```python
from build123d import *

# Parameters (mm, degrees)
BOSS_EXTRUDE2_DEPTH             = 6.896
SKETCH2_R                       = 1.7526
BOSS_EXTRUDE3_DEPTH             = 3.175
F_9_64_0_14063_DIAMETER_HOLE2_D = 3.572002
SKETCH9_W                       = 3.175
SKETCH9_H                       = 6.896
BOSS_EXTRUDE5_DEPTH             = 2.54
SKETCH10_W                      = 3.175
SKETCH10_H                      = 12.7
SKETCH10_W_2                    = 12.7
SKETCH10_H_2                    = 3.175
BOSS_EXTRUDE6_DEPTH             = 3.175
CUT_EXTRUDE1_DEPTH              = 97.085734956
CUT_EXTRUDE2_DEPTH              = 66.25004773
FILLET2_R                       = 1
CUT_EXTRUDE3_DEPTH              = 1


with BuildPart() as part:
    # Sketch1 → Boss-Extrude2 (new body)
    with BuildSketch(Plane(origin=(0, 0, 0), x_dir=(1, 0, 0), z_dir=(0, 1, 0))):
        with BuildLine():
            Line((12.363664128, -36.460798254), (6.35, -38.5))
            Line((6.35, -38.5), (-6.35, -38.5))
            Line((-6.35, -38.5), (-12.363664128, -36.460798254))
            ThreePointArc((-12.363664128, -36.460798254), (-27.097558937, -27.349082245), (-36.345013413, -12.7))
            ThreePointArc((-36.345013413, -12.7), (-37.940572846, -6.539337285), (-38.499480516, -0.2))
            Line((-38.499480516, -0.2), (-41.675, -0.2))
            Line((-41.675, -0.2), (-41.675, -15.875))
            Line((-41.675, -15.875), (-31.113215051, -27.726764582))
            ThreePointArc((-31.113215051, -27.726764582), (-23.009697223, -34.747078419), (-13.383265001, -39.467630318))
            Line((-13.383265001, -39.467630318), (-6.873668831, -41.675))
            Line((-6.873668831, -41.675), (6.873668831, -41.675))
            Line((6.873668831, -41.675), (13.383265001, -39.467630318))
            ThreePointArc((13.383265001, -39.467630318), (23.009697223, -34.747078419), (31.113215051, -27.726764582))
            Line((31.113215051, -27.726764582), (41.675, -15.875))
            Line((41.675, -15.875), (41.675, -0.2))
            Line((41.675, -0.2), (38.499480516, -0.2))
            ThreePointArc((38.499480516, -0.2), (37.940572846, -6.539337285), (36.345013413, -12.7))
            ThreePointArc((36.345013413, -12.7), (27.097558937, -27.349082245), (12.363664128, -36.460798254))
        make_face()
    extrude(amount=BOSS_EXTRUDE2_DEPTH)

    # Sketch2 → Boss-Extrude3 (add)
    with BuildSketch(Plane(origin=(41.675, 0, 0), x_dir=(0, 0, -1), z_dir=(1, 0, 0))):
        with BuildLine():
            Line((-15.875, 6.896), (-2.841859979, 17.12263896))
            ThreePointArc((-2.841859979, 17.12263896), (3.214674972, 17.143816898), (4.716891749, 11.27649989))
            Line((4.716891749, 11.27649989), (-0.2, 0))
            Line((-0.2, 0), (-0.2, 6.896))
            Line((-0.2, 6.896), (-15.875, 6.896))
        make_face()
        with Locations((0.2, 13.246)):
            Circle(SKETCH2_R, mode=Mode.SUBTRACT)
    boss_extrude3 = extrude(amount=-BOSS_EXTRUDE3_DEPTH)

    # Mirror1: Boss-Extrude3 across plane
    add(boss_extrude3.mirror(Plane.ZY))

    # 9/64 (0.14063) Diameter Hole2 (through all)
    with Locations(Plane.XY.offset(41.675)):
        with Locations((0, 3.448)):
            Hole(F_9_64_0_14063_DIAMETER_HOLE2_D / 2)

    # Sketch9 → Boss-Extrude5 (add)
    with BuildSketch(Plane.XY.offset(41.675)):
        with Locations((-5.0355, 3.448)):
            Rectangle(SKETCH9_W, SKETCH9_H)
        with Locations((5.0355, 3.448)):
            Rectangle(SKETCH9_W, SKETCH9_H)
    extrude(amount=BOSS_EXTRUDE5_DEPTH)

    # Sketch10 → Boss-Extrude6 (add)
    with BuildSketch(Plane(origin=(0, 0, 0), x_dir=(-1, 0, 0), z_dir=(0, -1, 0))):
        with Locations((40.0875, -7.545458209)):
            Rectangle(SKETCH10_W, SKETCH10_H)
        with Locations((-40.0875, -7.545458209)):
            Rectangle(SKETCH10_W, SKETCH10_H)
        with Locations((0, -40.0875)):
            Rectangle(SKETCH10_W_2, SKETCH10_H_2)
    extrude(amount=BOSS_EXTRUDE6_DEPTH)

    # Sketch11 → Cut-Extrude1 (cut, through all)
    with BuildSketch(Plane.ZY.offset(41.675)):
        Polygon((13.895458209, -0.4), (13.495458209, 0), (13.895458209, 0), align=None)
        Polygon((1.595458209, 0), (1.195458209, 0), (1.195458209, -0.4), align=None)
    extrude(amount=-CUT_EXTRUDE1_DEPTH, mode=Mode.SUBTRACT)

    # Sketch12 → Cut-Extrude2 (cut, through all)
    with BuildSketch(Plane.XY.offset(41.675)):
        Polygon((6.35, -0.4), (6.35, 0), (5.95, 0), align=None)
        Polygon((-5.95, 0), (-6.35, -0.4), (-6.35, 0), align=None)
    extrude(amount=-CUT_EXTRUDE2_DEPTH, mode=Mode.SUBTRACT)

    # Fillet2
    # the kernel refuses this fillet: 1 mm, written as the material it adds along each edge
    with BuildSketch(Plane(origin=(-38.5, 6.896, 0.2), x_dir=(1, 0, 0), z_dir=(0, 0, 1))) as fillet2_piece_1_section:
        with BuildLine():
            CenterArc((FILLET2_R, FILLET2_R), FILLET2_R, 180, 90)
            Line((0, FILLET2_R), (0, 0))
            Line((0, 0), (FILLET2_R, 0))
        make_face()
    fillet2_piece_1 = extrude(amount=18.175, mode=Mode.PRIVATE)
    fillet2_piece_1 = fillet2_piece_1 - Plane(origin=(0, 7.133182821, 0), x_dir=(-0.321134133185776, 0, 0.9470337208901384), z_dir=(0, -1, 0)) * Cylinder(38.5, 41, mode=Mode.PRIVATE)
    fillet2_piece_1 = split(fillet2_piece_1, bisect_by=Plane(origin=(-38.301679368, 10.067346027, 11.833340077), z_dir=(0, -0.7867194903062766, -0.617310654024562)), keep=Keep.TOP, mode=Mode.PRIVATE)
    add(fillet2_piece_1)
    with BuildSketch(Plane(origin=(38.5, 6.896, 0.2), x_dir=(-1, 0, 0), z_dir=(0, 0, 1))) as fillet2_piece_2_section:
        with BuildLine():
            CenterArc((FILLET2_R, -FILLET2_R), FILLET2_R, 90, 90)
            Line((0, -FILLET2_R), (0, 0))
            Line((0, 0), (FILLET2_R, 0))
        make_face()
    fillet2_piece_2 = extrude(amount=18.175, mode=Mode.PRIVATE)
    fillet2_piece_2 = fillet2_piece_2 - Plane(origin=(0, 7.133182807, 0), x_dir=(0.9999865069084622, 0, 0.0051948051948059485), z_dir=(0, -1, 0)) * Cylinder(38.5, 41, mode=Mode.PRIVATE)
    fillet2_piece_2 = split(fillet2_piece_2, bisect_by=Plane(origin=(38.301679263, 10.067346636, 11.833339301), z_dir=(0, -0.7867194903062766, -0.617310654024562)), keep=Keep.TOP, mode=Mode.PRIVATE)
    add(fillet2_piece_2)

    # Sketch14 → Cut-Extrude3 (cut)
    with BuildSketch(Plane(origin=(-38.5, 0, 0), x_dir=(0, 0, -1), z_dir=(1, 0, 0))):
        Polygon((-0.2, 0), (-0.2, 7.896), (3.242892532, 7.896), align=None)
    cut_extrude3 = extrude(amount=-CUT_EXTRUDE3_DEPTH, mode=Mode.SUBTRACT)

    # Mirror2: Cut-Extrude3 across plane
    add(cut_extrude3.mirror(Plane.ZY), mode=Mode.SUBTRACT)


solid = part.part
```
Design review of the part built by this model. Coordinates are the model's own, in mm. A direction names the side the tool comes from. Give positions to 0.01 mm unless a question says otherwise; leave off trailing zeros. Write each loop counter-clockwise with the first axis right and the second up, starting at its lowest first coordinate (ties: lowest second). Pieces come first, ordered by that corner, then holes. Notation, with made-up numbers: (-29.75, -26) -> (-1.75, -26) arc R21 cw to (-1.75, -15) -> close; hole circle Ø3 at (54.25, 1). An arc over 180 degrees is marked (long way). Answer in a Markdown table with one row per item.
(1) Consider section A-A (x = 0). State the section outline as (y, z) points (3 decimals).
Results:
| item | result |
|---|---|
| outline | (-3.175, 38.5) -> (1.662, 38.5) -> (1.662, 41.675) -> (-3.175, 41.675) -> close; (5.234, 38.5) -> (6.896, 38.5) -> (6.896, 41.675) -> (5.234, 41.675) -> close |
(2) To check wall thickness, follow probe 1 along Y at (x, z) = (-39, 0); probe 2 along X at (y, z) = (-1.5, 6.5) (3 decimals); probe 3 along Y at (x, z) = (0, 39.3) (3 decimals). State the ranges of each line that lie inside material, in increasing order.
Results:
| item | result |
|---|---|
| probe 1 | 7.9 to 11.5, 14.99 to 18.17 |
| probe 2 | -41.675 to -38.5, 38.5 to 41.675 |
| probe 3 | -3.175 to 1.662, 5.234 to 6.896 |
(3) Consider section B-B (z = 29). State the section outline as (x, y) points.
Results:
| item | result |
|---|---|
| outline | (-29.93, 0) -> (-25.32, 0) -> (-25.32, 6.9) -> (-29.93, 6.9) -> close; (25.32, 0) -> (29.93, 0) -> (29.93, 6.9) -> (25.32, 6.9) -> close |
(4) Mouldability with a two-part tool opening along X and no side actions: class faces 6 (the flat face through (-38.5, -2, 8)), 7 (the flat face through (-6.623, 3, 43)), 8 (the flat face through (-9.3, 3.4, 37.5)), 9 (the flat face through (-40.463, 5.717, -2.293)) as +X half, -X half, draft (parallel to the pull), parting line (faces both ways), or undercut.
Results:
| item | result |
|---|---|
| face 6 | undercut |
| face 7 | -X half |
| face 8 | undercut |
| face 9 | draft |
(5) Consider section D-D (x = 18.5). State the section outline as (y, z) points, then the cut area to 3 significant figures.
Results:
| item | result |
|---|---|
| outline | (0, 33.76) -> (6.9, 33.76) -> (6.9, 37.34) -> (0, 37.34) -> close |
| area | 24.7 mm2 |
(6) Clearance check with flat-ended pins moving along their axes: pin 1 (2 mm diameter, centred on y = 13.246, z = -0.2, fed in from -X); pin 2 (1.4 mm diameter, centred on y = -1, z = 39.5, fed in from -X); pin 3 (0.8 mm diameter, centred on x = 39, y = 5, fed in from -Z); pin 4 (1.4 mm diameter, centred on x = -39.5, y = -1.5, fed in from +Z). State where each tip first meets the part, or that it passes through.
Results:
| item | result |
|---|---|
| pin 1 | through |
| pin 2 | x = -6.35 |
| pin 3 | z = 0.2 |
| pin 4 | z = 13.9 |
(7) For faces 1 (the flat face through (6.35, -2, 40)), 2 (the flat face through (-3.448, 3, 43)), 3 (the flat face through (-39.5, 6, -1)), 4 (the flat face through (38.5, 12, 2)), 5 (the flat face through (38.5, -2, 8)), list the 3-axis set-ups (+Z, -Z, +X, -X, +Y, -Y) from which the entire face can be reached by the end or side of a thin tool; tool diameter is ignored.
Results:
| item | result |
|---|---|
| face 1 | +Z, -Z, +X, -Y |
| face 2 | +Z, +Y, -Y |
| face 3 | -Z, -Y |
| face 4 | +Z, -Z, +Y |
| face 5 | +Z, -Z, -Y |
(8) Consider section C-C (z = 6). State the section outline as (x, y) points (3 decimals), then the cut area to 3 significant figures.
Results:
| item | result |
|---|---|
| outline | (-41.675, -3.175) -> (-38.5, -3.175) -> (-38.5, 0) -> (-38.03, 0) -> (-38.03, 7.048) arc R1 cw to (-38.5, 7.896) -> (-38.5, 14.645) -> (-41.675, 14.645) -> close; (38.03, 0) -> (38.5, 0) -> (38.5, -3.175) -> (41.675, -3.175) -> (41.675, 14.645) -> (38.5, 14.645) -> (38.5, 7.896) arc R1 cw to (38.03, 7.048) -> close |
| area | 120 mm2 |
